from build123d import *

# Parameters (mm, degrees)
SKETCH_W     = 20
SKETCH_H     = 16
PAD_DEPTH    = 2
PAD001_DEPTH = 2
SKETCH004_R  = 1
PAD002_DEPTH = 3
SKETCH005_W  = 2
SKETCH005_H  = 1
PAD003_DEPTH = 2
PAD004_DEPTH = 2


with BuildPart() as part:
    # Sketch → Pad (new body)
    with BuildSketch(Plane.XZ):
        with Locations((10, 8)):
            Rectangle(SKETCH_W, SKETCH_H)
    extrude(amount=PAD_DEPTH)

    # Sketch001 (on Face6 of Pad) → Pad001 (join)
    with BuildSketch(Plane.XZ.offset(2)):
        with BuildLine():
            ThreePointArc((17.72495, 10.5), (17.610738, 13.825239), (14.497831, 15))
            ThreePointArc((5.497831, 15), (9.997831, 14.487175), (14.497831, 15))
            ThreePointArc((5.497831, 15), (2.18979, 13.514663), (2.728727, 9.928732))
            Line((9.5, 4), (2.728727, 9.928732))
            Line((9.5, 4), (9.5, 1))
            Line((9.5, 1), (11.5, 1))
            Line((11.5, 1), (11.5, 4))
            Line((11.5, 4), (17.72495, 10.5))
        make_face()
    extrude(amount=PAD001_DEPTH)

    # Sketch004 (on Face15 of Pad001) → Pad002 (join)
    with BuildSketch(Plane.XZ.offset(4)):
        with Locations((5, 12)):
            Circle(SKETCH004_R)
        with Locations((15, 12)):
            Circle(SKETCH004_R)
    extrude(amount=PAD002_DEPTH)

    # Sketch005 (on Face5 of Pad002) → Pad003 (join)
    with BuildSketch(Plane.XZ.offset(2)):
        with Locations((10.5, 0.5)):
            Rectangle(SKETCH005_W, SKETCH005_H)
    extrude(amount=PAD003_DEPTH)

    # Sketch006 (on Face12 of Pad003) → Pad004 (join)
    with BuildSketch(Plane(origin=(9.5, 0, 0), x_dir=(0, 0, -1), z_dir=(-1, 0, 0))):
        with BuildLine():
            Line((0, 2), (0, 4))
            ThreePointArc((0, 4), (6.989376, 11.448896), (-0.888889, 17.950464))
            ThreePointArc((-1, 19.944272), (-2.015402, 18.887686), (-0.888889, 17.950464))
            ThreePointArc((0, 2), (7.851742, 11.437563), (-1, 19.944272))
        make_face()
    extrude(amount=-PAD004_DEPTH)


solid = part.part
Source: CAD feature listing. Evaluate the final solid. Frame: model axes, mm. A direction names the side the tool comes from. Give positions to 0.01 mm unless a question says otherwise; leave off trailing zeros. Order: outer loops, then holes, each group sorted by start corner. A loop starts at its lowest first (then second) coordinate and runs counter-clockwise, first axis right, second up. Notation, with made-up numbers: (-9.5, 33) -> (48.5, 33) arc R21 ccw to (48.5, 46) -> close; hole circle Ø5 at (36, 43.5). An arc over 180 degrees is marked (long way). Write item = value, one per line.
Q1. Cut plane C-C, the plane z = -4. Output: boundary loops of the cut face in (x, y), and give its area (3 significant figures).
Data:
outline = (9.5, -18.33) -> (11.5, -18.33) -> (11.5, -16.75) -> (9.5, -16.75) -> close; (9.5, -5.25) -> (11.5, -5.25) -> (11.5, -3.54) -> (9.5, -3.54) -> close
area = 6.59 mm^2
Q2. Pin query (flat end, axial travel): pin 1 (1.6 mm diameter, centred on x = 4.5, z = 11.5, fed in from -Y); pin 2 (4 mm diameter, centred on y = -15.5, z = -2.5, fed in from +X); pin 3 (0.6 mm diameter, centred on x = 5, y = -1.5, fed in from -Z); pin 4 (2 mm diameter, centred on y = -5.5, z = 5.5, fed in from -X). Return the tip coordinate at first contact, or that it passes through.
Data:
pin_1 = -7
pin_2 = 11.5
pin_3 = 0
pin_4 = through
Q3. Cut plane B-B, the plane x = 8. Output: boundary loops of the cut face in (y, z), and give its area (3 significant figures).
Data:
outline = (-4, 5.31) -> (-2, 5.31) -> (-2, 0) -> (0, 0) -> (0, 16) -> (-2, 16) -> (-2, 14.59) -> (-4, 14.59) -> close
area = 50.5 mm^2
Q4. Pull-direction query (X, two-part tool) for faces 1 (the face through (10.486, -18.911, 2.016)), 2 (the face through (5, -5, 11)), 3 (the face through (11.5, -7.7, -6.4)); classes: released by +X, released by -X, zero draft, split by the parting line, or undercut.
Data:
face_1 = zero draft
face_2 = undercut
face_3 = released by +X
Q5. Material intervals for line 1 (Y direction, x = 13, z = 4.75); line 2 (Z direction, x = 2.25, y = -1); line 3 (Y direction, x = 12.25, z = 11.5), sorted ascending. Write a range as from..to.
Data:
line_1 = -2..0
line_2 = 0..16
line_3 = -4..0
Q6. Set-up query: faces 4 (the face through (9.934, -2.986, 14.487)), 5 (the face through (16, -5, 12)), 6 (the face through (9.5, -7.7, -6.4)). Return all of +Z, -Z, +X, -X, +Y, -Y with unobstructed straight access to the full face (end or side cutting, diameter ignored); none if empty.
Data:
face_4 = +Z, -Y
face_5 = -Y
face_6 = -Z, -X, -Y
Q7. Cut plane A-A, the plane z = 0.5. Output: boundary loops of the cut face in (x, y), and give its area (3 significant figures).
Data:
outline = (0, -2) -> (9.5, -2) -> (9.5, -4) -> (11.5, -4) -> (11.5, -2) -> (20, -2) -> (20, 0) -> (0, 0) -> close; (9.5, -19.92) -> (11.5, -19.92) -> (11.5, -17.99) -> (9.5, -17.99) -> close
area = 47.9 mm^2
Q8. Cut plane D-D, the plane z = 13.75. Output: boundary loops of the cut face in (x, y), and give its area (3 significant figures).
Data:
outline = (0, -2) -> (2.33, -2) -> (2.33, -4) -> (17.66, -4) -> (17.66, -2) -> (20, -2) -> (20, 0) -> (0, 0) -> close
area = 70.7 mm^2
